Input: part model. Units: mm. Frame: model coordinates. Give positions to 0.01 mm unless a question says otherwise; leave off trailing zeros. Loops run counter-clockwise (first coordinate to the right, second up) from the corner with the lowest first, then second, coordinate; pieces in that order, holes last. Notation, with made-up numbers: M -13,81.5 L 19,81.5 A20 cw 19,101.5 Z; hole C -28,0.5 d2. An arc over 180 degrees is marked long. Use a Markdown table: item, result. Add a question column.
Autodesk Inventor part; units mm, degrees
ref_plane "YZ Plane" through (0, 0, 0) normal (1, 0, 0) x (0, 1, 0)
ref_plane "XZ Plane" through (0, 0, 0) normal (0, 1, 0) x (-1, 0, 0)
ref_plane "XY Plane" through (0, 0, 0) normal (0, 0, 1) x (1, 0, 0)
sketch "スケッチ1" plane through (0, 0, 0) normal (0, 1, 0) x (-1, 0, 0)
  circle A0 centre (0, 0) radius 178.1675
  circle A1 centre (0, 0) radius 157.8276
  line L0 (168.1877, 0) -> (166.7488, -21.9529)
  line L1 (168.1877, 0) -> (130.1721, 2.4917) construction
  line L2 (249.4344, 0) -> (-249.4344, 0)
  line L3 (166.7488, -21.9529) -> (156.7702, -21.2989)
  line L4 (156.7702, -21.2989) -> (158.2091, 0.654) construction
  line L5 (158.2091, 0.654) -> (168.1877, 0)
  line L6 (157.4896, -10.3224) -> (0, 0)
  line L7 (166.7488, -21.9529) -> (162.4568, -43.5302)
  line L8 (162.4568, -43.5302) -> (152.649, -41.5793) construction
  line L9 (152.649, -41.5793) -> (156.9409, -20.002) construction
  line L10 (156.9409, -20.002) -> (166.7488, -21.9529) construction
  line L11 (162.4568, -43.5302) -> (155.3851, -64.3626)
  line L12 (155.3851, -64.3626) -> (145.9158, -61.1482) construction
  line L13 (145.9158, -61.1482) -> (152.9875, -40.3158) construction
  line L14 (152.9875, -40.3158) -> (162.4568, -43.5302) construction
  line L15 (155.3851, -64.3626) -> (145.6548, -84.0938)
  line L16 (145.6548, -84.0938) -> (136.6861, -79.6709) construction
  line L17 (136.6861, -79.6709) -> (146.4164, -59.9397) construction
  line L18 (146.4164, -59.9397) -> (155.3851, -64.3626) construction
  line L19 (0, 0) -> (111.6009, -111.6009)
  line L20 (145.6548, -84.0938) -> (137.3401, -78.5381) construction
  line L21 (137.3401, -78.5381) -> (125.1176, -96.8305) construction
  line L22 (125.1176, -96.8305) -> (133.4323, -102.3862) construction
  line L23 (133.4323, -102.3862) -> (145.6548, -84.0938)
  line L24 (133.4323, -102.3862) -> (125.9139, -95.7927) construction
  line L25 (125.9139, -95.7927) -> (111.4082, -112.3332) construction
  line L26 (111.4082, -112.3332) -> (118.9266, -118.9266)
  line L27 (118.9266, -118.9266) -> (133.4323, -102.3862)
  line L28 (111.6009, -111.6009) -> (118.9266, -118.9266)
  line L29 (166.7488, -21.9529) -> (176.7274, -22.6069) construction
  line L30 (118.9266, -118.9266) -> (125.9834, -125.9834)
  point P0 (154.795, -30.7906)
  point P1 (149.4517, -50.732)
  point P2 (141.5512, -69.8053)
  point P3 (131.2288, -87.6843)
  point P4 (118.661, -104.0629)
  point P5 (157.8276, 0)
  point P6 (178.1675, 0)
  dimension "d0" = 22
  dimension "d1" = 10
  dimension "d2" = 45
  dimension "d4" = 315.6551
extrude "押し出し1" add sketch "スケッチ1" along normal blind 5.5 contours L30 L27 L23 L15 L11 L7 L0 L2 A0 | L28 A1 L2 L0 L7 L11 L15 L23 L27
sketch "スケッチ2" plane through (0, 5.5, 0) normal (0, 1, 0) x (1, 0, 0)
  circle A0 centre (0, 0) radius 309.8276
  line L0 (-168.1877, 0) -> (-166.7488, 21.9529)
  line L1 (-166.7488, 21.9529) -> (-162.4568, 43.5302)
  line L2 (-162.4568, 43.5302) -> (-155.3851, 64.3626)
  line L3 (-155.3851, 64.3626) -> (-145.6548, 84.0938)
  line L4 (-133.4323, 102.3862) -> (-145.6548, 84.0938)
  line L5 (-118.9266, 118.9266) -> (-133.4323, 102.3862)
  line L6 (-167.4682, 10.9764) -> (-166.0294, 32.9293)
  line L7 (-166.0294, 32.9293) -> (-275.7938, 40.1237)
  line L8 (-275.7938, 40.1237) -> (-277.2327, 18.1708)
  line L9 (-277.2327, 18.1708) -> (-167.4682, 10.9764)
  line L10 (-164.6028, 32.7415) -> (-160.3108, 54.3188)
  line L11 (-160.3108, 54.3188) -> (-268.1972, 75.7787)
  line L12 (-268.1972, 75.7787) -> (-272.4892, 54.2015)
  line L13 (-272.4892, 54.2015) -> (-164.6028, 32.7415)
  circle A1 centre (-166.7488, 21.9529) radius 11
  circle A2 centre (-162.4568, 43.5302) radius 11
  line L14 (-158.921, 53.9464) -> (-151.8493, 74.7789)
  line L15 (-151.8493, 74.7789) -> (-256.0116, 110.1372)
  line L16 (-256.0116, 110.1372) -> (-263.0833, 89.3047)
  line L17 (-263.0833, 89.3047) -> (-158.921, 53.9464)
  circle A3 centre (-155.3851, 64.3626) radius 11
  arc A4 (-275.7591, 62.4834) -> (-281.3553, 41.7349) centre (-166.7488, 21.9529) ccw
  line L18 (-178.1663, 0.654) -> (-158.2091, -0.654)
  line L19 (-158.2091, -0.654) -> (-156.7702, 21.2989)
  line L20 (-156.7702, 21.2989) -> (-176.7274, 22.6069)
  line L21 (-176.7274, 22.6069) -> (-178.1663, 0.654)
  line L22 (-177.4468, 11.6305) -> (-275.7938, 40.1237)
  line L23 (-176.7274, 22.6069) -> (-176.008, 33.5834)
  line L24 (-176.008, 33.5834) -> (-275.7591, 62.4834)
  line L25 (-275.7938, 40.1237) -> (-281.3553, 41.7349)
  circle A5 centre (0, 0) radius 137.8276
  line L26 (0, 0) -> (-219.0812, 219.0812)
  line L27 (-111.6009, 111.6009) -> (-125.9834, 125.9834)
  line L28 (-433.7586, 0) -> (433.7586, 0)
  circle A6 centre (0, 0) radius 279.8276 construction
  arc A7 (-111.6009, 111.6009) -> (-157.8276, 0) centre (0, 0) ccw
  point P0 (-158.1662, 0)
  point P1 (-137.8276, 0)
  point P2 (-97.4588, 97.4588)
  point P3 (-309.8276, 0)
  dimension "d7" = 22
  dimension "d10" = 20
  dimension "d11" = 100
  dimension "d12" = 30
  dimension "d14" = 20
  dimension "d17" = 122
extrude "押し出し2" add sketch "スケッチ2" against normal blind 5.5 contours L26 L5 L4 L3 A3 L15 L16 L17 A2 L11 L12 L24 A4 L25 L8 L9 L21 L18 L28 A0 | L18 L21 L9 L0 | L0 A1 L19 L28 | A5 L28 A7 A1 A2 A3 L26 | L26 A7 A3 L3 L4 L5 | A1 L21 L20 L0 | L9 L21 A1 | L0 L20 L19 A1 | L19 A7 L28 | L6 A1 L1 | L20 L23 A1 L6 | L1 A1 A7 L19 L20 | L22 L7 L23 A1 L21 | L9 L8 L22 | A1 L23 L21 | A1 A7 L19 | A7 A3 L2 L3 | A3 A7 | A2 L10 L1 | A1 L7 L24 L13 | A2 A7 A1 | L13 L24 L12 L11 A2 | L1 L2 A2 A7 | A1 L23 L7 | L25 A4 L24 L12 L13 L7 | A7 A1 | A7 A2 A3 | L3 L14 A3 | L10 A2 L2 | L13 L12 L24 | A7 A2 | A3 L14 L2 | L17 L16 L15 A3
sketch "スケッチ3" plane through (0, 5.5, 0) normal (0, 1, 0) x (1, 0, 0)
  circle A0 centre (0, 0) radius 157.8276
  arc A1 (-97.4588, 97.4588) -> (-137.8276, 0) centre (0, 0) ccw
  line L0 (-97.4588, 97.4588) -> (-219.0812, 219.0812)
  line L1 (-309.8276, 0) -> (-137.8276, 0)
  arc A2 (-219.0812, 219.0812) -> (-309.8276, 0) centre (0, 0) ccw
  point P0 (-157.8276, 0)
  point P1 (-111.6009, 111.6009)
  dimension "d18" = 20
extrude "押し出し3" cut sketch "スケッチ3" against normal through all contours A0 L1 A2 L0
sketch "スケッチ4" plane through (0, 5.5, 0) normal (0, 1, 0) x (1, 0, 0)
  line L0 (-152.8276, 9.2) -> (-142.8276, 9.2)
  line L1 (-142.8276, 9.2) -> (-142.8276, 12.2)
  line L2 (-142.8276, 12.2) -> (-152.8276, 12.2)
  line L3 (-152.8276, 12.2) -> (-152.8276, 9.2)
  line L4 (-149.3276, 5.7) -> (-146.3276, 5.7)
  line L5 (-146.3276, 5.7) -> (-146.3276, 15.7)
  line L6 (-146.3276, 15.7) -> (-149.3276, 15.7)
  line L7 (-149.3276, 15.7) -> (-149.3276, 5.7)
  line L8 (-157.8276, 0) -> (-137.8276, 0)
  line L9 (-97.4588, 97.4588) -> (-111.6009, 111.6009)
  line L10 (-104.5299, 104.5299) -> (-123.5496, 85.5102) construction
  line L11 (-109.621, 92.3676) -> (-107.4997, 94.489)
  line L12 (-107.4997, 94.489) -> (-114.5708, 101.56)
  line L13 (-114.5708, 101.56) -> (-116.6921, 99.4387)
  line L14 (-116.6921, 99.4387) -> (-109.621, 92.3676)
  line L15 (-116.6921, 94.489) -> (-114.5708, 92.3676)
  line L16 (-114.5708, 92.3676) -> (-107.4997, 99.4387)
  line L17 (-107.4997, 99.4387) -> (-109.621, 101.56)
  line L18 (-109.621, 101.56) -> (-116.6921, 94.489)
  line L19 (-97.4588, 97.4588) -> (-111.6009, 111.6009)
  line L20 (-108.5604, 93.4283) -> (-115.6315, 100.4994) construction
  point P0 (0, 0)
  point P1 (-147.8276, 0)
  point P2 (-147.8276, 5.7)
  point P3 (-147.8276, 9.2)
  point P4 (-149.3276, 10.7)
  point P5 (-152.8276, 10.7)
  point P6 (-147.8276, 0)
  point P7 (-149.3276, 12.2)
  point P8 (-149.3276, 9.2)
  point P9 (-146.3276, 9.2)
  point P10 (-146.3276, 12.2)
  point P11 (-108.5604, 100.4994)
  point P12 (-113.1566, 98.0245)
  point P13 (-111.0353, 98.0245)
  point P14 (-114.2172, 96.9638)
  point P15 (-112.0959, 94.8425)
  point P16 (-109.9746, 96.9638)
  point P17 (-112.0959, 99.0852)
  dimension "d21" = 10
  dimension "d22" = 3
  dimension "d23" = 5.7
  dimension "d30" = 5.7
extrude "押し出し4" cut sketch "スケッチ4" against normal through all
equation "\"d30\" = d23"
properties part number "back_under" material "木材 (カエデ材)"
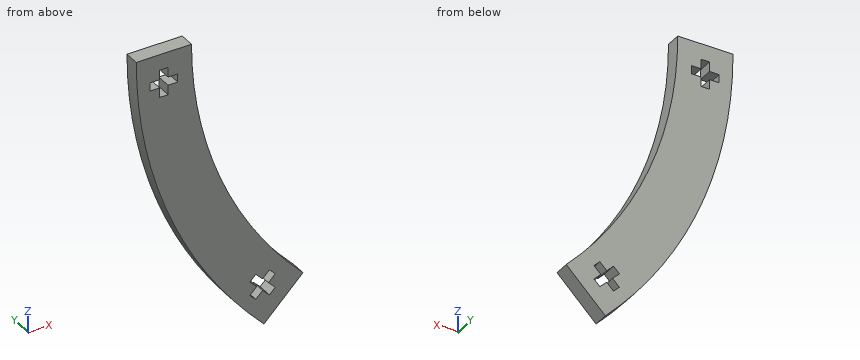
1) Section query D-D, the plane z = -38. Return the cut outline in (x, y), and give its area (3 significant figures).
2) Section query B-B, the plane z = -7.5. Return the cut outline in (x, y), and give its area (3 significant figures).
3) Ray query, line 1 (X direction, y = 1.85, z = -15); line 2 (X direction, y = 4.4, z = -95); line 3 (X direction, y = 4.2, z = -89). Return the intervals inside material, ascending. Write a range as [from, to].
4) Section query C-C, the plane x = -105. Return the cut outline in (y, z), and give its area (3 significant figures).
5) Section query A-A, the plane y = 2.25. Return the cut outline in (x, z).
6) Contact query for flat-ended pins moving along their axis: P1, Ø1.8, axis at y = 4, z = -13.5, coming from the +X side; P2, Ø3, axis at y = 3.5, z = -56, coming from the -X side; P3, Ø3, axis at x = -144, y = 2.5, coming from the -Z side. Output: stop coordinate, or through.
Entries:
| question | item | result |
|---|---|---|
| 1 | outline | M -153.18,0 L -132.49,0 L -132.49,5.5 L -153.18,5.5 Z |
| 1 | area | 114 mm² |
| 2 | outline | M -157.65,0 L -149.33,0 L -149.33,5.5 L -157.65,5.5 Z; M -146.33,0 L -137.62,0 L -137.62,5.5 L -146.33,5.5 Z |
| 2 | area | 93.6 mm² |
| 3 | line 1 | x = [-157.11, -149.33], [-146.33, -137.01] |
| 3 | line 2 | x = [-126.03, -116.18], [-108.01, -99.86] |
| 3 | line 3 | x = [-130.34, -105.24] |
| 4 | outline | M 0,-105 L 5.5,-105 L 5.5,-89.28 L 0,-89.28 Z |
| 4 | area | 86.4 mm² |
| 5 | outline | M -157.83,0 A157.83 ccw -111.6,-111.6 L -97.46,-97.46 A137.83 cw -137.83,0 Z; hole M -152.83,-12.2 L -149.33,-12.2 L -149.33,-15.7 L -146.33,-15.7 L -146.33,-12.2 L -142.83,-12.2 L -142.83,-9.2 L -146.33,-9.2 L -146.33,-5.7 L -149.33,-5.7 L -149.33,-9.2 L -152.83,-9.2 Z; hole M -116.69,-99.44 L -114.57,-101.56 L -112.1,-99.09 L -109.62,-101.56 L -107.5,-99.44 L -109.97,-96.96 L -107.5,-94.49 L -109.62,-92.37 L -112.1,-94.84 L -114.57,-92.37 L -116.69,-94.49 L -114.22,-96.96 Z |
| 6 | P1 | stops at x = -137.07 |
| 6 | P2 | stops at x = -148.12 |
| 6 | P3 | stops at z = -67.85 |
